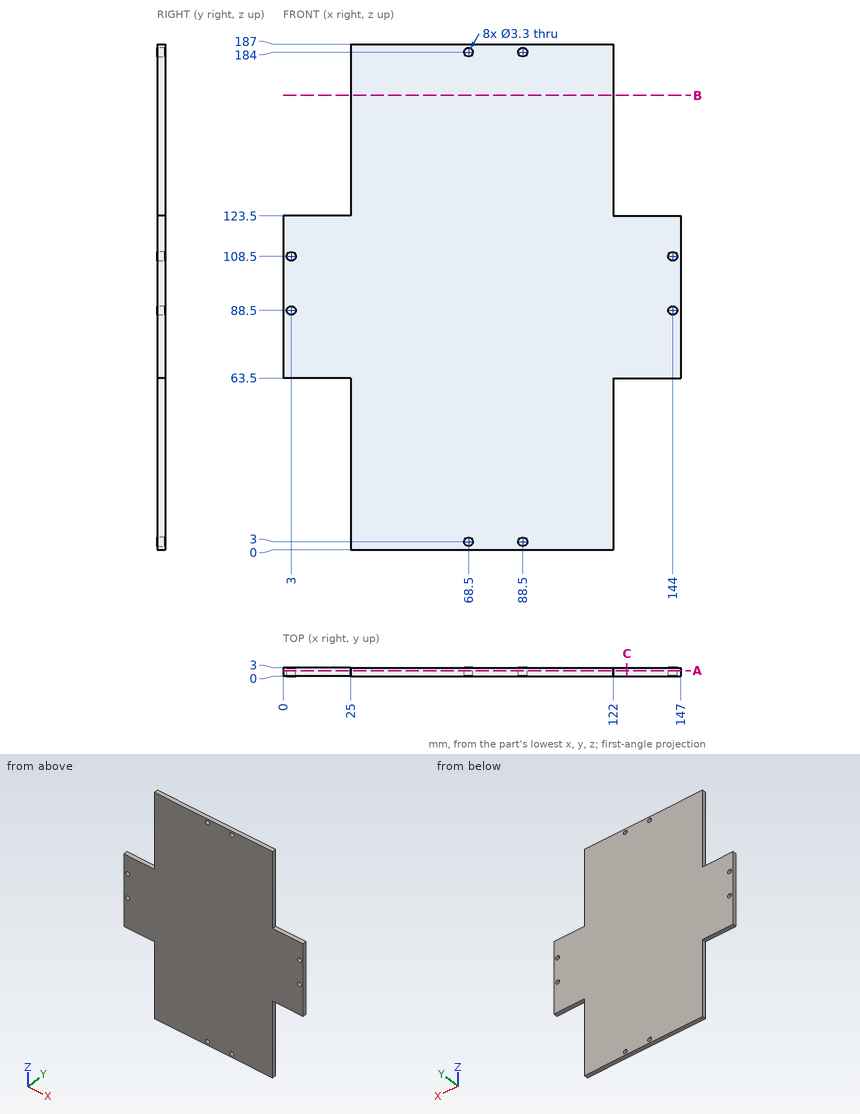
Source: three-view drawing plus pictorial views. Frame: mm from the lowest corner of the part. Coordinates: 2 decimals unless noted, no trailing zeros. Order: outer loops, then holes, each group sorted by start corner. A loop starts at its lowest first (then second) coordinate and runs counter-clockwise, first axis right, second up.
Item 1: First-contact query: P1, Ø0.9, axis at y = 1.5, z = 47.5, coming from the -X side; P2, Ø0.9, axis at x = 15, y = 1, coming from the -Z side; P3, Ø0.9, axis at y = 1, z = 41.5, coming from the +X side. Flat tips, straight axial feed; report the tip coordinate or a pass-through.
Output values:
P1: stops at x = 25
P2: stops at z = 63.5
P3: stops at x = 122
Item 2: Cut plane A-A (y = 2). Count the separate pieces of the cut face and the enclosed holes in it, plus the area to 3 significant figures.
Output values:
separate pieces: 1
enclosed holes: 8
area: 21,100 mm2
Item 3: Cut plane B-B (z = 168). Return loops of the section in (x, y), plus the area to 3 significant figures.
Output values:
outline: (25, 0) - (122, 0) - (122, 3) - (25, 3) - close
area: 291 mm2
Item 4: Cut plane C-C (x = 127). Return loops of the section in (y, z), plus the area to 3 significant figures.
Output values:
outline: (0, 63.5) - (3, 63.5) - (3, 123.5) - (0, 123.5) - close
area: 180 mm2
Item 5: Material intervals for line 1 (Z direction, x = 3, y = 2.45); line 2 (X direction, y = 0.75, z = 3); line 3 (Z direction, x = 88.5, y = 2), sorted ascending.
Output values:
line 1: z = 63.5 to 86.85, 90.15 to 106.85, 110.15 to 123.5
line 2: x = 25 to 66.85, 70.15 to 86.85, 90.15 to 122
line 3: z = 0 to 1.35, 4.65 to 182.35, 185.65 to 187
